For this review, take the finished solid that the model builds, in its own axes (mm). A direction names the side the tool comes from. Round coordinates to 2 decimals unless told otherwise and drop trailing zeros. Order: outer loops, then holes, each group sorted by start corner. A loop starts at its lowest first (then second) coordinate and runs counter-clockwise, first axis right, second up.
from build123d import *

# Parameters (mm, degrees)
SKETCH1_W           = 86
SKETCH1_H           = 20
BOSS_EXTRUDE1_DEPTH = 1.3
SKETCH2_W           = 30
SKETCH2_H           = 1.4
SKETCH2_W_2         = 1.4
SKETCH2_H_2         = 10
BOSS_EXTRUDE2_DEPTH = 1.3
CUT_EXTRUDE1_DEPTH  = 46.858586982
SKETCH4_W           = 1
SKETCH4_H           = 10
CUT_EXTRUDE2_DEPTH  = 46.858586982
CUT_EXTRUDE3_DEPTH  = 46.858586982


with BuildPart() as part:
    # Sketch1 → Boss-Extrude1 (new body)
    with BuildSketch(Plane.XY):
        Rectangle(SKETCH1_W, SKETCH1_H)
    extrude(amount=BOSS_EXTRUDE1_DEPTH)

    # Sketch2 → Boss-Extrude2 (add)
    with BuildSketch(Plane.XY.offset(1.3)):
        with Locations((0, -10.7)):
            Rectangle(SKETCH2_W, SKETCH2_H)
        with Locations((-43.7, 3.5)):
            Rectangle(SKETCH2_W_2, SKETCH2_H_2)
        with Locations((43.7, 3.5)):
            Rectangle(SKETCH2_W_2, SKETCH2_H_2)
    extrude(amount=-BOSS_EXTRUDE2_DEPTH)

    # Sketch3 → Cut-Extrude1 (cut, through all)
    with BuildSketch(Plane.XY.offset(1.3)):
        with BuildLine():
            Line((-34, 10), (34, 10))
            ThreePointArc((34, 10), (0, 4.033829384), (-34, 10))
        make_face()
    extrude(amount=-CUT_EXTRUDE1_DEPTH, mode=Mode.SUBTRACT)

    # Sketch4 → Cut-Extrude2 (cut, through all)
    with BuildSketch(Plane.XY.offset(1.3)):
        with Locations((-10.5, -3)):
            Rectangle(SKETCH4_W, SKETCH4_H)
        with Locations((10.5, -3)):
            Rectangle(SKETCH4_W, SKETCH4_H)
    extrude(amount=-CUT_EXTRUDE2_DEPTH, mode=Mode.SUBTRACT)

    # Sketch5 → Cut-Extrude3 (cut, through all)
    with BuildSketch(Plane.XY.offset(1.3)):
        Polygon((-37.347292806, 4.71481035), (-37.347292806, -2.961858542), (-32.708450107, -2.961858542), (-32.708450107, 0.938053462), align=None)
        Polygon((32.708450107, -2.961858542), (32.708450107, 0.938053462), (37.347292806, 4.71481035), (37.347292806, -2.961858542), align=None)
    extrude(amount=-CUT_EXTRUDE3_DEPTH, mode=Mode.SUBTRACT)


solid = part.part
(1) Add section C-C on y = 7.75. Give the boundary of the cut face in (x, z).
(2) Tool access review of faces 1 (the face through (-1, -1, 1.3)), 2 (the face through (34.995, 2.8, 0.659)): name each direction out of +Z, -Z, +X, -X, +Y, -Y from which nothing blocks a thin tool from reaching the whole face with its end or side.
(3) Wall thickness on L1, parallel to X at y = -5.25, z = 0.45; L2, parallel to X at y = -2.5, z = 0.6; L3, parallel to Y at x = -36.5, z = 0.5: over which ranges is each line inside the solid? List them lowest first.
(4) Add section D-D on x = 1.5. Give the boundary of the cut face in (y, z).
(5) Draft analysis for pull direction Y (two halves, no side actions). For faces 3 (the face through (0.486, 4.035, 0.659)), 4 (the face through (-1, -1, 0)), 5 (the face through (-34.995, 2.8, 0.659)), state which applies: pulls with the +Y half, pulls with the -Y half, needs draft (parallel to the pull), parting line crosses it, or undercut.
(6) Add section A-A on y = -4.5. Give the boundary of the cut face in (x, z), plus the area to 3 significant figures.
(7) Add section B-B on z = 0.75. Count the separate pieces of the cut face and the enclosed holes in it, plus the area to 3 significant figures.
Here are the results:
1. outline: (-44.4, 0) - (-26.99, 0) - (-26.99, 1.3) - (-44.4, 1.3) - close; (26.99, 0) - (44.4, 0) - (44.4, 1.3) - (26.99, 1.3) - close
2. face 1: +Z, +X, -X, +Y, -Y
2. face 2: +Z, -Z
3. L1: x = -43 to -11, -10 to 10, 11 to 43
3. L2: x = -43 to -37.35, -32.71 to -11, -10 to 10, 11 to 32.71, 37.35 to 43
3. L3: y = -10 to -2.96, 4.02 to 10
4. outline: (-11.4, 0) - (4.05, 0) - (4.05, 1.3) - (-11.4, 1.3) - close
5. face 3: pulls with the +Y half
5. face 4: needs draft
5. face 5: undercut
6. outline: (-43, 0) - (-11, 0) - (-11, 1.3) - (-43, 1.3) - close; (-10, 0) - (10, 0) - (10, 1.3) - (-10, 1.3) - close; (11, 0) - (43, 0) - (43, 1.3) - (11, 1.3) - close
6. area: 109 mm2
7. separate pieces: 1
7. enclosed holes: 4
7. area: 1,440 mm2
